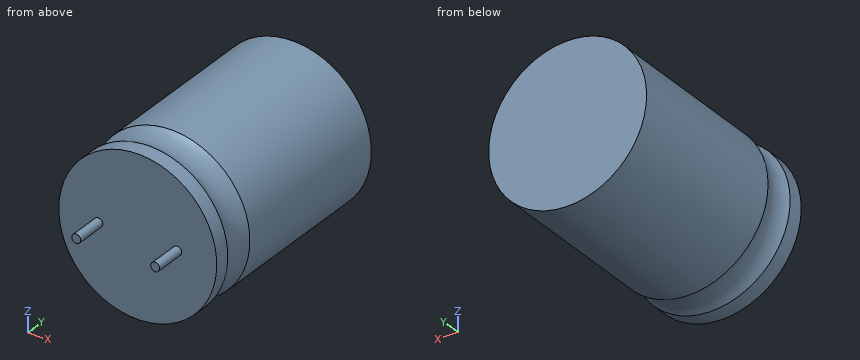
from build123d import *

# Parameters (mm, degrees)
SKETCH2_R           = 0.282946128
BOSS_EXTRUDE1_DEPTH = 2


with BuildPart() as part:
    # Sketch1 → Revolve1 (revolve)
    with BuildSketch(Plane.XY, mode=Mode.PRIVATE) as revolve1_sk:
        with BuildLine():
            Line((0, 14), (0, 0))
            Line((0, 0), (5, 0))
            Line((5, 0), (5, 1))
            ThreePointArc((5, 1), (4.732050808, 2), (5, 3))
            Line((5, 3), (5, 14))
            Line((5, 14), (0, 14))
        make_face()
    revolve(revolve1_sk.sketch.rotate(Axis((0, 14, 0), (0, -1, 0)), 180), axis=Axis((0, 14, 0), (0, -1, 0)))

    # Sketch2 → Boss-Extrude1 (add)
    with BuildSketch(Plane.XZ):
        with Locations(Location((2.5, 0, 0), (0, 0, 180))):
            Circle(SKETCH2_R)
        with Locations(Location((-2.5, 0, 0), (0, 0, 180))):
            Circle(SKETCH2_R)
    extrude(amount=BOSS_EXTRUDE1_DEPTH)


solid = part.part
Can you work these out from the model? Positions are in its coordinate system, mm. Give positions to 0.01 mm unless a question says otherwise; leave off trailing zeros. Loops run counter-clockwise (first coordinate to the right, second up) from the corner with the lowest first, then second, coordinate; pieces in that order, holes last. Notation, with made-up numbers: M 83,4.25 L 140,4.25 A13 ccw 140,21.25 Z; hole C 53,29 d11. An arc over 180 degrees is marked long. One line per item, written item: value. Start each with the question number.
1) If I drill on line 1 (Y direction, x = 0, z = 4); line 2 (X direction, y = 1.5, z = -2.25); line 3 (X direction, y = 0.75, z = 2), over which ranges is the centre line in solid material (lowest first)? Write a range as [from, to].
2) I'm going to push flat-ended pins straight in: pin 1 (1.5 mm diameter, centred on y = 2, z = -3.5, fed in from -X); pin 2 (2 mm diameter, centred on y = 6.5, z = 1.5, fed in from +X); pin 3 (1 mm diameter, centred on x = 2, z = 2.5, fed in from -Y). Where does each tip first touch, or does it pass through?
3) If we section it at C-C, the plane y = 11: Write out the boundary of the cut face in (x, z), and give its area (3 significant figures).
4) If we section it at B-B, the plane z = 0: Write out the boundary of the cut face in (x, y), and give its area (3 significant figures).
5) If we section it at A-A, the plane x = 0: Write out the boundary of the cut face in (y, z).
Completed:
1. line 1: y = [0, 14]
1. line 2: x = [-4.23, 4.23]
1. line 3: x = [-4.58, 4.58]
2. pin 1: stops at x = -3.85
2. pin 2: stops at x = 4.97
2. pin 3: stops at y = 0
3. outline: C 0,0 d10
3. area: 78.5 mm^2
4. outline: M -5,0 L -2.78,0 L -2.78,-2 L -2.22,-2 L -2.22,0 L 2.22,0 L 2.22,-2 L 2.78,-2 L 2.78,0 L 5,0 L 5,1 A2 cw 5,3 L 5,14 L -5,14 L -5,3 A2 cw -5,1 Z
4. area: 142 mm^2
5. outline: M 0,-5 L 1,-5 A2 cw 3,-5 L 14,-5 L 14,5 L 3,5 A2 cw 1,5 L 0,5 Z
